Source: CAD feature listing. Evaluate the final solid. Frame: model axes, mm. Coordinates: 2 decimals unless noted, no trailing zeros. Order: outer loops, then holes, each group sorted by start corner. A loop starts at its lowest first (then second) coordinate and runs counter-clockwise, first axis right, second up. Notation, with made-up numbers: (19.25, 43.5) - (33.25, 43.5) arc R36 cw to (33.25, 79.5) - close; hole circle Ø2 at (49, 59.5). An arc over 180 degrees is marked (long way). One line per question, with ' | ' between items.
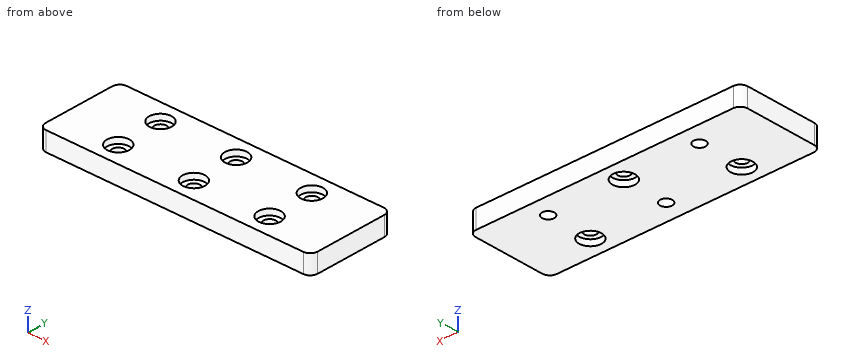
from build123d import *

# Parameters (mm, degrees)
F1_W     = 182.603597641
F1_H     = 58.2040771842
F3_DEPTH = 12.7
F2_R     = 4.06875
F4_DEPTH = 12.701
F5_R     = 7.5
F6_DEPTH = 4
F7_R     = 7.5
F8_DEPTH = 4
F9_R     = 5


with BuildPart() as f3:
    # F1 (on Top) → F3 (new body)
    with BuildSketch(Plane.XY):
        Rectangle(F1_W, F1_H)
    extrude(amount=F3_DEPTH)

    # F2 (on Top) → F4 (cut, through all)
    with BuildSketch(Plane.XY):
        with Locations((-50.8, 15.3108183295)):
            Circle(F2_R)
        with Locations((0, 15.3108183295)):
            Circle(F2_R)
        with Locations((50.8, 15.3108183295)):
            Circle(F2_R)
        with Locations((50.8, -15.2709130198)):
            Circle(F2_R)
        with Locations((0, -15.2709130198)):
            Circle(F2_R)
        with Locations((-50.8, -15.2709130198)):
            Circle(F2_R)
    extrude(amount=F4_DEPTH, mode=Mode.SUBTRACT)

    # F5 (on face) → F6 (cut)
    with BuildSketch(Plane.XY.offset(12.7)):
        with Locations((-50.8, 15.3108183295)):
            Circle(F5_R)
        with Locations((0, -15.2709130198)):
            Circle(F5_R)
        with Locations((50.8, 15.3108183295)):
            Circle(F5_R)
        with Locations((-50.8, -15.2709130198)):
            Circle(F5_R)
        with Locations((0, 15.3108183295)):
            Circle(F5_R)
        with Locations((50.8, -15.2709130198)):
            Circle(F5_R)
    extrude(amount=-F6_DEPTH, mode=Mode.SUBTRACT)

    # F7 (on face) → F8 (cut)
    with BuildSketch(Plane(origin=(0, 0, 0), x_dir=(1, 0, 0), z_dir=(0, 0, -1))):
        with Locations((0, -15.3108183295)):
            Circle(F7_R)
        with Locations((-50.8, 15.2709130198)):
            Circle(F7_R)
        with Locations((50.8, 15.2709130198)):
            Circle(F7_R)
    extrude(amount=-F8_DEPTH, mode=Mode.SUBTRACT)

    # F9
    f9_edges = [f3.edges().sort_by_distance(p)[0] for p in [
        (-91.301799, -29.102039, 6.35),
        (-91.301799, 29.102039, 6.35),
        (91.301799, 29.102039, 6.35),
        (91.301799, -29.102039, 6.35),
    ]]
    fillet(f9_edges, radius=F9_R)


solid = f3.part
(1) Pin query (flat end, axial travel): P1, Ø9, axis at x = 50.8, y = -15.27, coming from the -Z side; P2, Ø12, axis at x = 2, y = 13, coming from the +Z side; P3, Ø9, axis at x = 50.8, y = 15.31, coming from the +Z side. Return the tip coordinate at first contact, or that it passes through.
Taken from the geometry:
P1: stops at z = 4 | P2: stops at z = 12.7 | P3: stops at z = 8.7
(2) Cut plane B-B (z = 1.75). Return the cut outline in (x, y).
Taken from the geometry:
outline: (-91.3, -24.1) arc R5 ccw to (-86.3, -29.1) - (86.3, -29.1) arc R5 ccw to (91.3, -24.1) - (91.3, 24.1) arc R5 ccw to (86.3, 29.1) - (-86.3, 29.1) arc R5 ccw to (-91.3, 24.1) - close; hole circle Ø15 at (-50.8, -15.27); hole circle Ø8.14 at (-50.8, 15.31); hole circle Ø15 at (0, 15.31); hole circle Ø8.14 at (0, -15.27); hole circle Ø15 at (50.8, -15.27); hole circle Ø8.14 at (50.8, 15.31)
(3) Material intervals for L1, parallel to Y at x = -50.8, z = 5; L2, parallel to X at y = -16, z = 8; L3, parallel to Y at x = 50.8, z = 3, sorted ascending. Write a range as from..to.
Taken from the geometry:
L1: y = -29.1..-19.34, -11.2..11.24, 19.38..29.1 | L2: x = -91.3..-54.8, -46.8..-4, 4..46.8, 54.8..91.3 | L3: y = -29.1..-22.77, -7.77..11.24, 19.38..29.1
(4) Cut plane A-A (x = -50.8). Return the cut outline in (y, z), and give its area (3 significant figures).
Taken from the geometry:
outline: (-29.1, 0) - (-22.77, 0) - (-22.77, 4) - (-19.34, 4) - (-19.34, 8.7) - (-22.77, 8.7) - (-22.77, 12.7) - (-29.1, 12.7) - close; (-11.2, 4) - (-7.77, 4) - (-7.77, 0) - (11.24, 0) - (11.24, 8.7) - (7.81, 8.7) - (7.81, 12.7) - (-7.77, 12.7) - (-7.77, 8.7) - (-11.2, 8.7) - close; (19.38, 0) - (29.1, 0) - (29.1, 12.7) - (22.81, 12.7) - (22.81, 8.7) - (19.38, 8.7) - close | area: 450 mm²
